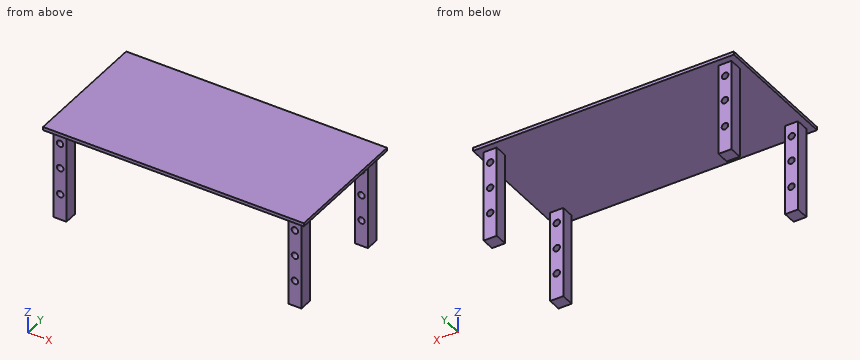
from build123d import *

# Parameters (mm, degrees)
F0_W     = 2000
F0_H     = 1000
F1_DEPTH = 25
F2_W     = 98.425484
F2_H     = 100
F3_DEPTH = 700
F4_W     = 100
F4_H     = 100
F5_DEPTH = 700
F6_W     = 100
F6_H     = 100
F7_DEPTH = 700
F8_W     = 100
F8_H     = 100
F9_DEPTH = 700
F11_D    = 50
F13_D    = 50
F15_D    = 50
F17_D    = 50
F19_D    = 50
F21_D    = 50


with BuildPart() as f1:
    # F0 (on Top) → F1 (new body)
    with BuildSketch(Plane.XY):
        with Locations((0, -62.883471)):
            Rectangle(F0_W, F0_H)
    extrude(amount=F1_DEPTH)

    # F2 (on face) → F3 (join)
    with BuildSketch(Plane(origin=(0, 0, 0), x_dir=(1, 0, 0), z_dir=(0, 0, -1))):
        with Locations((-900.787258, 462.883471)):
            Rectangle(F2_W, F2_H)
    extrude(amount=F3_DEPTH)

    # F4 (on face) → F5 (join)
    with BuildSketch(Plane(origin=(0, 0, 0), x_dir=(1, 0, 0), z_dir=(0, 0, -1))):
        with Locations((-900, -337.116529)):
            Rectangle(F4_W, F4_H)
    extrude(amount=F5_DEPTH)

    # F6 (on face) → F7 (join)
    with BuildSketch(Plane(origin=(0, 0, 0), x_dir=(1, 0, 0), z_dir=(0, 0, -1))):
        with Locations((900, -337.116529)):
            Rectangle(F6_W, F6_H)
    extrude(amount=F7_DEPTH)

    # F8 (on face) → F9 (join)
    with BuildSketch(Plane(origin=(0, 0, 0), x_dir=(1, 0, 0), z_dir=(0, 0, -1))):
        with Locations((900, 462.883471)):
            Rectangle(F8_W, F8_H)
    extrude(amount=F9_DEPTH)

    # F11 (through all)
    with Locations(Plane.XZ.offset(512.883471)):
        with Locations((-900, -500.001549)):
            Hole(F11_D / 2)

    # F13 (through all)
    with Locations(Plane.XZ.offset(512.883471)):
        with Locations((-900, -293.510616)):
            Hole(F13_D / 2)

    # F15 (through all)
    with Locations(Plane.XZ.offset(512.883471)):
        with Locations((-901.574516, -100)):
            Hole(F15_D / 2)

    # F17 (through all)
    with Locations(Plane.XZ.offset(512.883471)):
        with Locations((900, -500)):
            Hole(F17_D / 2)

    # F19 (through all)
    with Locations(Plane.XZ.offset(512.883471)):
        with Locations((900, -300)):
            Hole(F19_D / 2)

    # F21 (through all)
    with Locations(Plane.XZ.offset(512.883471)):
        with Locations((900, -100)):
            Hole(F21_D / 2)


solid = f1.part
Read the model definition and answer for the solid it produces. Units are mm, in the model's axes. Round coordinates to 2 decimals unless told otherwise and drop trailing zeros. Write each loop counter-clockwise with the first axis right and the second up, starting at its lowest first coordinate (ties: lowest second). Pieces come first, ordered by that corner, then holes.
1. Given pin 1 Ø4 at (x, y) = (-118.5, -381) entering from -Z, flat-ended and moving along its own axis, determine where the tip first touches the part or whether it passes through.
2. The part is cut by section A-A, the plane z = -628. Determine the outline of the cut face in (x, y).
3. The part is cut by section B-B, the plane z = -100. State how many separate pieces and enclosed holes the cut face has, then the cut area to 3 significant figures.
4. The part is cut by section D-D, the plane y = 315.5. Determine the outline of the cut face in (x, z).
5. Straight lines are drawn through the part: L1, parallel to Z at x = 900, y = 347; L2, parallel to X at y = 328, z = -484; L3, parallel to Z at x = 83, y = -512.5. For each, find the intervals that lie inside material, in ascending order.
Values:
1. pin 1: stops at z = 0
2. outline: (-950, -512.88) - (-851.57, -512.88) - (-851.57, -412.88) - (-950, -412.88) - close; (-950, 287.12) - (-850, 287.12) - (-850, 387.12) - (-950, 387.12) - close; (850, -512.88) - (950, -512.88) - (950, -412.88) - (850, -412.88) - close; (850, 287.12) - (950, 287.12) - (950, 387.12) - (850, 387.12) - close
3. separate pieces: 8
3. enclosed holes: 0
3. area: 19,800 mm2
4. outline: (-1000, 0) - (-950, 0) - (-950, -700) - (-850, -700) - (-850, 0) - (850, 0) - (850, -700) - (950, -700) - (950, 0) - (1000, 0) - (1000, 25) - (-1000, 25) - close; hole circle Ø50 at (-901.57, -100); hole circle Ø50 at (-900, -500); hole circle Ø50 at (-900, -293.51); hole circle Ø50 at (900, -500); hole circle Ø50 at (900, -300); hole circle Ø50 at (900, -100)
5. L1: z = -700 to -525, -475 to -325, -275 to -125, -75 to 25
5. L2: x = -950 to -919.21, -880.79 to -850, 850 to 880.79, 919.21 to 950
5. L3: z = 0 to 25
